Verification items for this drawing (mm, ordinates from the low corner). Coordinates: 2 decimals unless noted, no trailing zeros. Loops run counter-clockwise (first coordinate to the right, second up) from the corner with the lowest first, then second, coordinate; pieces in that order, holes last. Notation, with made-up numbers: (73, -35.75) - (77, -35.75) arc R19 cw to (77, -6.75) - close; hole circle Ø7 at (8, 27). An arc over 180 degrees is marked (long way). One line per item, written item: value. Start each with the question number.
(1) Section check D-D (y = 27). Record the boundary of the cut face in (x, z), plus the area to 3 significant figures.
(2) Draft check along Z on the marked faces 1, 2 and 3. Enter one of: +Z half, -Z half, draft (parallel to the pull), parting line (faces both ways), or undercut.
(3) Section check B-B (y = 7). Record the boundary of the cut face in (x, z), plus the area to 3 significant figures.
(4) Section check C-C (x = 32). Record the boundary of the cut face in (y, z).
(5) Section check A-A (z = 7.5). Record the boundary of the cut face in (x, y), plus the area to 3 significant figures.
(6) Thickness scan on probe 1 along Y at (x, z) = (13, 10.25); probe 2 along X at (y, z) = (25.5, 4.75); probe 3 along X at (y, z) = (26, 3.75). Record the ranges inside material, lowest first. Write a range as [from, to].
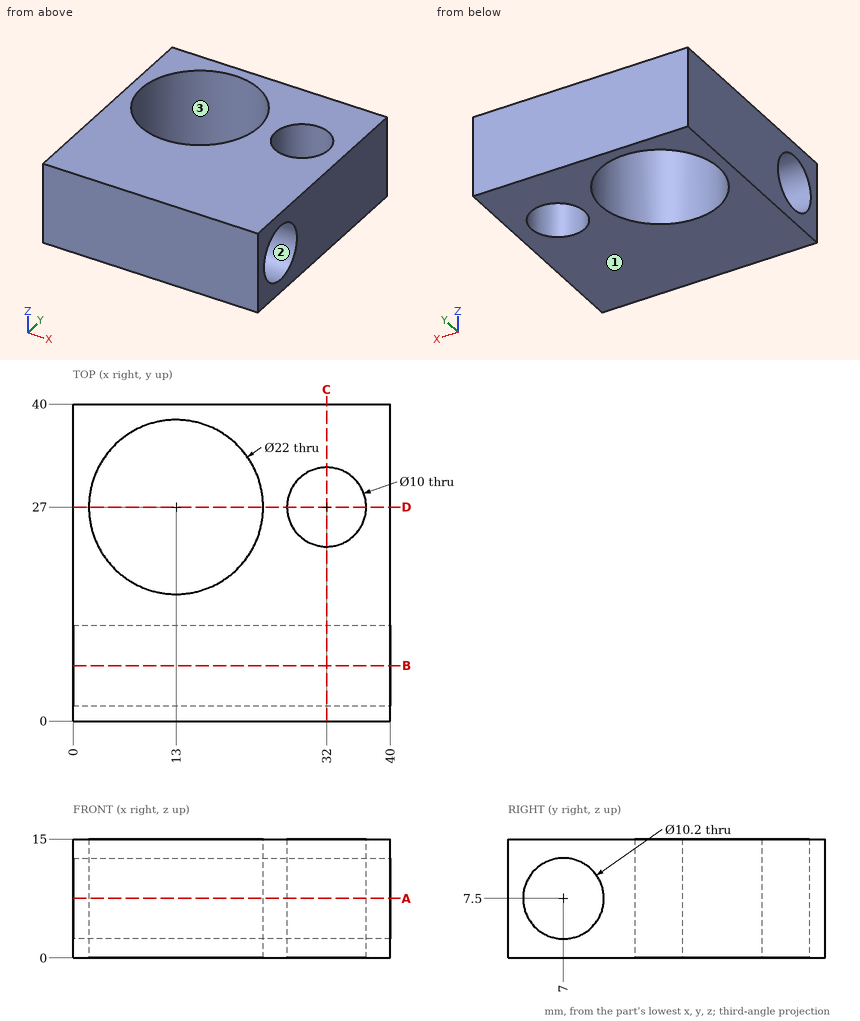
Responses:
1. outline: (0, 0) - (2, 0) - (2, 15) - (0, 15) - close; (24, 0) - (27, 0) - (27, 15) - (24, 15) - close; (37, 0) - (40, 0) - (40, 15) - (37, 15) - close
1. area: 120 mm²
2. face 1: -Z half
2. face 2: undercut
2. face 3: draft
3. outline: (0, 0) - (40, 0) - (40, 2.4) - (0, 2.4) - close; (0, 12.6) - (40, 12.6) - (40, 15) - (0, 15) - close
3. area: 192 mm²
4. outline: (0, 0) - (22, 0) - (22, 15) - (0, 15) - close; (32, 0) - (40, 0) - (40, 15) - (32, 15) - close; hole circle Ø10.2 at (7, 7.5)
5. outline: (0, 0) - (40, 0) - (40, 1.9) - (0, 1.9) - close; (0, 12.1) - (40, 12.1) - (40, 40) - (0, 40) - close; hole circle Ø22 at (13, 27); hole circle Ø10 at (32, 27)
5. area: 733 mm²
6. probe 1: y = [0, 2.7], [11.3, 16], [38, 40]
6. probe 2: x = [0, 2.1], [23.9, 27.23], [36.77, 40]
6. probe 3: x = [0, 2.05], [23.95, 27.1], [36.9, 40]
